Work out the finished part from the listing and answer in its coordinate system (mm). A direction names the side the tool comes from. Coordinates: 2 decimals unless noted, no trailing zeros. Order: outer loops, then holes, each group sorted by start corner. A loop starts at its lowest first (then second) coordinate and runs counter-clockwise, first axis right, second up. Notation, with made-up numbers: M 22,-31.75 L 70,-31.75 A37 ccw 70,5.25 Z; hole C -35.5,-22 d1. An arc over 180 degrees is marked long. Use a Markdown table: item, result.
Autodesk Fusion 360 part; units mm, degrees
sketch "Sketch1" plane through (0, 0, 0) normal (0, 0, 1) x (1, 0, 0)
  circle A0 centre (0, 0) radius 75
extrude "Extrude1" add sketch "Sketch1" along normal blind 10
sketch "Sketch2" plane through (0, 0, 0) normal (0, 0, 1) x (1, 0, 0)
  circle A0 centre (0, 0) radius 69.6419
  circle A1 centre (0, 0) radius 63.2456
extrude "Extrude2" add sketch "Sketch2" against normal blind 5
sketch "Sketch3" plane through (0, 0, 0) normal (0, 0, 1) x (1, 0, 0)
  line L0 (-40, 50) -> (-35, 50)
  line L1 (-40, 50) -> (-37.5, 50)
  line L2 (40, 50) -> (-40, 50)
  line L3 (-37.5, 50) -> (-10, 0)
  line L4 (-10, 0) -> (-40, -50)
  line L5 (-40, -50) -> (40, -50)
  line L6 (40, -50) -> (10, 0)
  line L7 (40, 55) -> (10, 0)
extrude "Extrude3" add 1 faces at (67.2505, -3.4599, -5) along direction (0, 0, 1) blind 5
extrude "Extrude4" add sketch "Sketch3" against normal blind 10
sketch "Sketch4" plane through (0, 0, 0) normal (0, 0, 1) x (1, 0, 0)
1. Section A-A on x = 0 is taken. Determine the outline of the cut face in (y, z), then the cut area to 3 significant figures.
Answers below:
| item | result |
|---|---|
| outline | M -75,0 L -69.64,0 L -69.64,-5 L -63.25,-5 L -63.25,0 L -50,0 L -50,-10 L 50,-10 L 50,0 L 63.25,0 L 63.25,-5 L 69.64,-5 L 69.64,0 L 75,0 L 75,10 L -75,10 Z |
| area | 2,560 mm² |
2. For faces 4 (the face through (2.18, 63.21, -2.46)), 5 (the face through (-9.764, -74.362, 4.93)), determine the directions among +Z, -Z, +X, -X, +Y, -Y from which every point of the face is accessible in a straight line to the end or side of a thin tool.
Answers below:
| item | result |
|---|---|
| face 4 | -Z |
| face 5 | +Z, -Z |
3. Section B-B on z = -7.25 is taken. Determine the outline of the cut face in (x, y).
Answers below:
| item | result |
|---|---|
| outline | M -40,-50 L 40,-50 L 10,0 L 37.27,50 L -37.5,50 L -10,0 Z |
4. For a pull along X with two mould halves and no side action, classify faces 1 (the face through (-1, 1, 10)), 2 (the face through (66.426, 20.919, -2.465)), 3 (the face through (-1, -50, -5)) as +X half, -X half, draft (parallel to the pull), parting line (faces both ways), or undercut.
Answers below:
| item | result |
|---|---|
| face 1 | draft |
| face 2 | parting line |
| face 3 | undercut |
5. Flat-ended cylindrical pins translate along their axes: P1, Ø2, axis at y = 1.5, z = 8, coming from the -X side; P2, Ø1, axis at x = -35, z = 8, coming from the -Y side; P3, Ø3, axis at x = -1, z = -5, coming from the +Y side. Find the tip coordinate at first contact, or state that the pin passes through.
Answers below:
| item | result |
|---|---|
| P1 | x = -75 |
| P2 | y = -66.59 |
| P3 | y = 69.64 |
6. Section D-D on x = 32.5 is taken. Determine the outline of the cut face in (y, z), then the cut area to 3 significant figures.
Answers below:
| item | result |
|---|---|
| outline | M -67.59,0 L -61.59,0 L -61.59,-5 L -54.26,-5 L -54.26,0 L -50,0 L -50,-10 L -37.5,-10 L -37.5,0 L 41.25,0 L 41.25,-10 L 50,-10 L 50,0 L 54.26,0 L 54.26,-5 L 61.59,-5 L 61.59,0 L 67.59,0 L 67.59,10 L -67.59,10 Z |
| area | 1,640 mm² |
7. Section C-C on y = -10.5 is taken. Determine the outline of the cut face in (x, z).
Answers below:
| item | result |
|---|---|
| outline | M -74.26,0 L -68.85,0 L -68.85,-5 L -62.37,-5 L -62.37,0 L -16.3,0 L -16.3,-10 L 16.3,-10 L 16.3,0 L 62.37,0 L 62.37,-5 L 68.85,-5 L 68.85,0 L 74.26,0 L 74.26,10 L -74.26,10 Z |
8. Find the intervals of material crossed by probe 1 along Y at (x, z) = (-34, -0.25); probe 2 along X at (y, z) = (-47.5, -1); probe 3 along X at (y, z) = (-1, 5), in increasing order.
Answers below:
| item | result |
|---|---|
| probe 1 | -60.78 to -53.33, -50 to -40, 43.64 to 50, 53.33 to 60.78 |
| probe 2 | -50.93 to -41.76, -38.5 to 38.5, 41.76 to 50.93 |
| probe 3 | -74.99 to 74.99 |
